```python
from build123d import *

# Parameters (mm, degrees)
F1_DEPTH = 10
F2_R     = 1.75
F3_DEPTH = 15.001
F5_DEPTH = 5.001


# Not quite as in the source:
# - a feature names something its author has since deleted; it is built from what else it names


with BuildPart() as f1:
    # F0 (on Front) → F1 (new body)
    with BuildSketch(Plane.XZ):
        Polygon((31.7108153552, 10), (201.7108153552, 10), (201.7108153552, 15), (30.3418431431, 15), (26.0328800881, 15), (19.6614095846, 5), (10.3393448517, 5), (10.3393448517, 0), (25.3393448517, 0), align=None)
    extrude(amount=F1_DEPTH)

    # F2 (on face) → F3 (cut, through all)
    with BuildSketch(Plane.XY.offset(15)):
        with Locations((118.7108153552, -5)):
            Circle(F2_R)
        with Locations((124.7108153552, -5)):
            Circle(F2_R)
        with Locations((196.7108153552, -5)):
            Circle(F2_R)
    extrude(amount=-F3_DEPTH, mode=Mode.SUBTRACT)

    # F4 (on face) → F5 (cut, through all)
    with BuildSketch(Plane.XY.offset(5)):
        with BuildLine():
            ThreePointArc((13.2503772181, -5), (15.0003772181, -6.75), (16.7503772181, -5))
            ThreePointArc((16.7503772181, -5), (15.0003772181, -3.25), (13.2503772181, -5))
        make_face()
    extrude(amount=-F5_DEPTH, mode=Mode.SUBTRACT)


solid = f1.part
```
Model file for the job. Use its own axes, mm. A direction names the side the tool comes from. Round coordinates to 2 decimals unless told otherwise and drop trailing zeros. Order: outer loops, then holes, each group sorted by start corner. A loop starts at its lowest first (then second) coordinate and runs counter-clockwise, first axis right, second up. Notation, with made-up numbers: (23, 67) -> (50, 67) arc R26 cw to (50, 106) -> close; hole circle Ø5 at (26, 36.25). An arc over 180 degrees is marked (long way). Use one line per item in the form item = value.
Item 1: Cut at C-C, the plane x = 163. Write the cut outline in (y, z), and give its area (3 significant figures).
Returned:
outline = (-10, 10) -> (0, 10) -> (0, 15) -> (-10, 15) -> close
area = 50.0 mm^2
Item 2: Pull direction Y, two halves, no side cores. Call faces 1 (the face through (126.38, -4.47, 12.54)), 2 (the face through (10.339, -5, 3)), 3 (the face through (98, 0, 11)): released by +Y, released by -Y, zero draft, split by the parting line, or undercut.
Returned:
face_1 = undercut
face_2 = zero draft
face_3 = released by +Y
Item 3: Flat gauge pins, fed straight in: pin 1 Ø3 at (x, y) = (16.5, -4.5) entering from +Z; pin 2 Ø4 at (x, y) = (118.71, -5) entering from -Z; pin 3 Ø5 at (x, y) = (125.5, -4.5) entering from +Z. Where does each tip first touch, or does it go through?
Returned:
pin_1 = 5
pin_2 = 10
pin_3 = 15
Item 4: Drill centre lines: line 1 (X direction, y = -6, z = 12); line 2 (Z direction, x = 32.5, y = -3); line 3 (X direction, y = -4.5, z = 12.5). Where is each one in solid material? Low to high.
Returned:
line_1 = 24.12 to 117.27, 120.15 to 123.27, 126.15 to 195.27, 198.15 to 201.71
line_2 = 10 to 15
line_3 = 24.44 to 117.03, 120.39 to 123.03, 126.39 to 195.03, 198.39 to 201.71
Item 5: Cut at B-B, the plane z = 13.25. Write the cut outline in (x, y), and give its area (3 significant figures).
Returned:
outline = (24.92, -10) -> (201.71, -10) -> (201.71, 0) -> (24.92, 0) -> close; hole circle Ø3.5 at (118.71, -5); hole circle Ø3.5 at (124.71, -5); hole circle Ø3.5 at (196.71, -5)
area = 1,740 mm^2
Item 6: Tool access for faces 4 (the face through (115, -5, 15)), 5 (the face through (116, -5, 10)), 6 (the face through (17, -5, 5)): list every direction of +Z, -Z, +X, -X, +Y, -Y with a clear straight run to the whole face (end or side of a thin tool).
Returned:
face_4 = +Z, +X, -X, +Y, -Y
face_5 = -Z, +X, +Y, -Y
face_6 = +Z, -X, +Y, -Y
Item 7: Cut at D-D, the plane z = 3. Write the cut outline in (x, y).
Returned:
outline = (10.34, -10) -> (27.25, -10) -> (27.25, 0) -> (10.34, 0) -> close; hole circle Ø3.5 at (15, -5)
Item 8: Cut at A-A, the plane y = -5. Write the cut outline in (x, z), and give its area (3 significant figures).
Returned:
outline = (10.34, 0) -> (13.25, 0) -> (13.25, 5) -> (10.34, 5) -> close; (16.75, 0) -> (25.34, 0) -> (31.71, 10) -> (116.96, 10) -> (116.96, 15) -> (26.03, 15) -> (19.66, 5) -> (16.75, 5) -> close; (120.46, 10) -> (122.96, 10) -> (122.96, 15) -> (120.46, 15) -> close; (126.46, 10) -> (194.96, 10) -> (194.96, 15) -> (126.46, 15) -> close; (198.46, 10) -> (201.71, 10) -> (201.71, 15) -> (198.46, 15) -> close
area = 944 mm^2
